Geometry: see drawing. Coordinates: mm, zero at the bounding-box minimum. A direction names the side the tool comes from. Coordinates: 2 decimals unless noted, no trailing zeros. Write each loop counter-clockwise with the first axis right and the second up, starting at its lowest first coordinate (ties: lowest second). Pieces come first, ordered by that corner, then holes.
1) Section query B-B (y = 10.25). Output: boundary loops of the cut face in (x, z).
2) Draft query along X for the marked faces 1, 2 and 3. Return one class per face: pulls with the +X half, pulls with the -X half, needs draft (parallel to the pull), parting line crosses it, or undercut.
3) Section query D-D (x = 65). Output: boundary loops of the cut face in (y, z), then the cut area to 3 significant figures.
4) Pin query (flat end, axial travel): pin 1 Ø4.5 at (x, y) = (5, 5) entering from +Z; pin 2 Ø6 at (x, y) = (55, 6) entering from +Z; pin 3 Ø4 at (x, z) = (51, 6.5) entering from +Y. Return the tip coordinate at first contact, or that it passes through.
5) Line query: L1, parallel to X at y = 4, z = 6; L2, parallel to X at y = 6, z = 6.5; L3, parallel to Y at x = 67.5, z = 3.25. Output: solid intervals per line, ascending.
6) Section query A-A (z = 5.25). Output: boundary loops of the cut face in (x, y).
7) Set-up query: the marked faces 4 and 5. Return all of +Z, -Z, +X, -X, +Y, -Y with unobstructed straight access to the full face (end or side cutting, diameter ignored); none if empty.
8) Section query C-C (x = 43). Output: boundary loops of the cut face in (y, z), then the cut area to 3 significant figures.
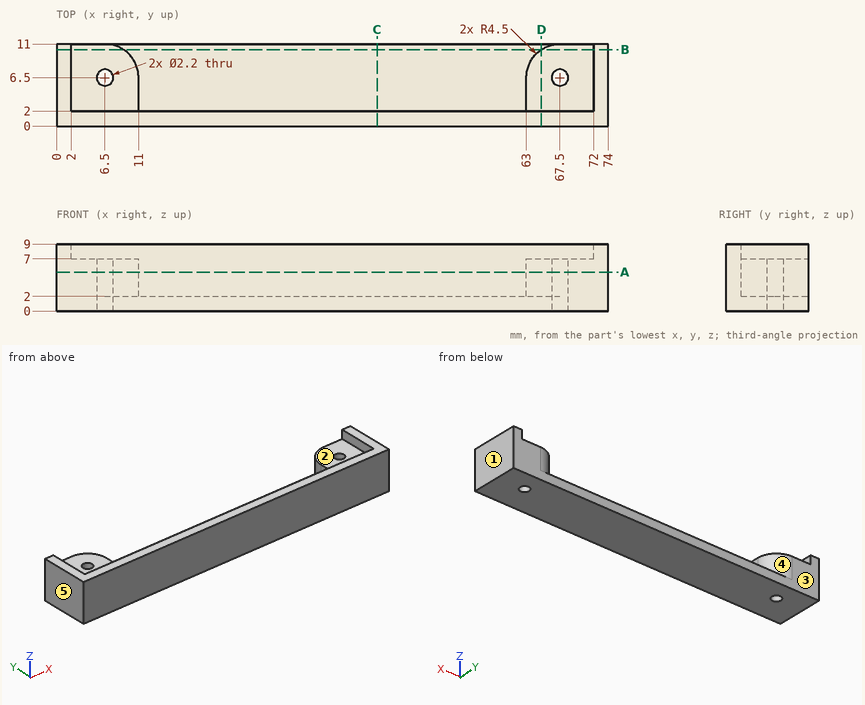
Answer:
1. outline: (0, 0) - (74, 0) - (74, 9) - (72, 9) - (72, 7) - (65.01, 7) - (65.01, 2) - (8.99, 2) - (8.99, 7) - (2, 7) - (2, 9) - (0, 9) - close
2. face 1: pulls with the +X half
2. face 2: undercut
2. face 3: needs draft
3. outline: (0, 0) - (11, 0) - (11, 2) - (10.24, 2) - (10.24, 7) - (2, 7) - (2, 9) - (0, 9) - close
3. area: 77.2 mm2
4. pin 1: stops at z = 7
4. pin 2: stops at z = 2
4. pin 3: stops at y = 2
5. L1: x = 0 to 11, 63 to 74
5. L2: x = 0 to 5.52, 7.48 to 11, 63 to 66.52, 68.48 to 74
5. L3: y = 0 to 5.4, 7.6 to 11
6. outline: (0, 0) - (74, 0) - (74, 11) - (67.5, 11) arc R4.5 ccw to (63, 6.5) - (63, 2) - (11, 2) - (11, 6.5) arc R4.5 ccw to (6.5, 11) - (0, 11) - close; hole circle Ø2.2 at (6.5, 6.5); hole circle Ø2.2 at (67.5, 6.5)
7. face 4: +Z, +Y
7. face 5: +Z, -Z, -X, +Y, -Y
8. outline: (0, 0) - (11, 0) - (11, 2) - (2, 2) - (2, 9) - (0, 9) - close
8. area: 36.0 mm2
